Geometry check sheet. Reference: the model listing, model coordinates, mm. A direction names the side the tool comes from. Round coordinates to 2 decimals unless told otherwise and drop trailing zeros. Order: outer loops, then holes, each group sorted by start corner. A loop starts at its lowest first (then second) coordinate and runs counter-clockwise, first axis right, second up.
(1) Material ranges on line 1 along Z through (x, y) = (-2.5, -0.75); line 2 along Z through (x, y) = (-0.75, -3.5); line 3 along Z through (x, y) = (3.75, 2), recorded low to high.
(2) Go/stop test with flat-tipped pins: pin 1 (2 mm diameter, centred on x = 3.5, y = -2, fed in from -Z); pin 2 (1 mm diameter, centred on y = -2, z = -1, fed in from +X). Record where each tip stops, or that it passes through.
(3) Sectioned sample at C-C (z = 1.15). Record the boundary of the cut face in (x, y), plus the area to 3 significant figures.
(4) Sectioned sample at A-A (x = 0). Record the boundary of the cut face in (y, z) (3 decimals), plus the area to 3 significant figures.
(5) Release check for a two-part mould opening along Z. For faces 1 (the face through (0, 0, 2.55)), 2 (the face through (-2.5, 1.917, -0.394)), 3 (the face through (0, 4, 0.5)) record: +Z half, -Z half, draft (parallel to the pull), parting line (faces both ways), or undercut.
(6) Sectioned sample at B-B (y = 0). Record the boundary of the cut face in (x, z) (3 decimals).
(7) Set-up check for faces 4 (the face through (-3.2, -0.9, 0)), 5 (the face through (4.75, -0.08, 0.25)), 6 (the face through (-3.796, 0.167, 1.141)): record each of +Z, -Z, +X, -X, +Y, -Y from which the full face is reachable in a straight line by a thin tool's end or side.
from build123d import *

# Parameters (mm, degrees)
F0_R      = 4.75
F1_DEPTH  = 0.5
F2_R      = 3.8
F3_DEPTH  = 1.3
F4_R      = 4.175
F4_R_2    = 3.8
F5_DEPTH  = 0.75
F6_SIZE   = 0.5
F8_DEPTH  = 2.551
F9_R      = 3.15
F10_DEPTH = 0.8
F11_R     = 2.165
F12_DEPTH = 1.67
F13_R     = 3.14
F14_DEPTH = 0.67
F15_SIZE  = 0.5


with BuildPart() as f1:
    # F0 (on Top) → F1 (new body)
    with BuildSketch(Plane.XY):
        Circle(F0_R)
    extrude(amount=F1_DEPTH)

    # F2 (on face) → F3 (join)
    with BuildSketch(Plane.XY.offset(0.5)):
        Circle(F2_R)
    extrude(amount=F3_DEPTH)

    # F4 (on face) → F5 (join)
    with BuildSketch(Plane.XY.offset(1.8)):
        Circle(F4_R)
        Circle(F4_R_2, mode=Mode.SUBTRACT)
        Circle(F4_R_2)
    extrude(amount=F5_DEPTH)

    # F6
    f6_edges = [f1.edges().sort_by_distance(p)[0] for p in [
        (-4.175, 0, 2.55),
    ]]
    chamfer(f6_edges, length=F6_SIZE)

    # F7 (on face) → F8 (cut, through all)
    with BuildSketch(Plane(origin=(0, 0, 0), x_dir=(1, 0, 0), z_dir=(0, 0, -1))):
        with BuildLine():
            Line((-1.9965971051, 4.31), (0, 4.31))
            Line((0, 4.31), (1.9965971051, 4.31))
            ThreePointArc((1.9965971051, 4.31), (0, 4.75), (-1.9965971051, 4.31))
        make_face()
        with BuildLine():
            Line((0, -4.31), (-1.9965971051, -4.31))
            ThreePointArc((-1.9965971051, -4.31), (0, -4.75), (1.9965971051, -4.31))
            Line((1.9965971051, -4.31), (0, -4.31))
        make_face()
    extrude(amount=-F8_DEPTH, mode=Mode.SUBTRACT)

    # F9 (on face) → F10 (join)
    with BuildSketch(Plane(origin=(0, 0, 0), x_dir=(1, 0, 0), z_dir=(0, 0, -1))):
        Circle(F9_R)
    extrude(amount=F10_DEPTH)

    # F11 (on face) → F12 (join)
    with BuildSketch(Plane(origin=(0, 0, -0.8), x_dir=(1, 0, 0), z_dir=(0, 0, -1))):
        Circle(F11_R)
    extrude(amount=F12_DEPTH)

    # F13 (on face) → F14 (join)
    with BuildSketch(Plane(origin=(0, 0, -2.47), x_dir=(1, 0, 0), z_dir=(0, 0, -1))):
        Circle(F13_R)
    extrude(amount=F14_DEPTH)

    # F15
    f15_edges = [f1.edges().sort_by_distance(p)[0] for p in [
        (-3.14, 0, -3.14),
    ]]
    chamfer(f15_edges, length=F15_SIZE)


solid = f1.part
Answer below:
1. line 1: z = -3.14 to -2.47, -0.8 to 2.55
1. line 2: z = 0 to 2.55
1. line 3: z = 0 to 0.5
2. pin 1: stops at z = -2.75
2. pin 2: stops at x = 2.75
3. outline: circle Ø7.6 at (0, 0)
3. area: 45.4 mm2
4. outline: (-4.31, 0) - (-3.15, 0) - (-3.15, -0.8) - (-2.165, -0.8) - (-2.165, -2.47) - (-3.14, -2.47) - (-3.14, -2.64) - (-2.64, -3.14) - (2.64, -3.14) - (3.14, -2.64) - (3.14, -2.47) - (2.165, -2.47) - (2.165, -0.8) - (3.15, -0.8) - (3.15, 0) - (4.31, 0) - (4.31, 0.5) - (3.8, 0.5) - (3.8, 1.8) - (4.175, 1.8) - (4.175, 2.05) - (3.675, 2.55) - (-3.675, 2.55) - (-4.175, 2.05) - (-4.175, 1.8) - (-3.8, 1.8) - (-3.8, 0.5) - (-4.31, 0.5) - close
4. area: 36.4 mm2
5. face 1: +Z half
5. face 2: draft
5. face 3: undercut
6. outline: (-4.75, 0) - (-3.15, 0) - (-3.15, -0.8) - (-2.165, -0.8) - (-2.165, -2.47) - (-3.14, -2.47) - (-3.14, -2.64) - (-2.64, -3.14) - (2.64, -3.14) - (3.14, -2.64) - (3.14, -2.47) - (2.165, -2.47) - (2.165, -0.8) - (3.15, -0.8) - (3.15, 0) - (4.75, 0) - (4.75, 0.5) - (3.8, 0.5) - (3.8, 1.8) - (4.175, 1.8) - (4.175, 2.05) - (3.675, 2.55) - (-3.675, 2.55) - (-4.175, 2.05) - (-4.175, 1.8) - (-3.8, 1.8) - (-3.8, 0.5) - (-4.75, 0.5) - close
7. face 4: -Z
7. face 5: +Z, -Z, +X
7. face 6: none
